Job drawing, mm, ordinate dimensions from the low corner. One solid piece. A direction names the side the tool comes from. Coordinates: 2 decimals unless noted, no trailing zeros. Write each loop counter-clockwise with the first axis right and the second up, starting at its lowest first coordinate (ties: lowest second). Pieces come first, ordered by that corner, then holes.
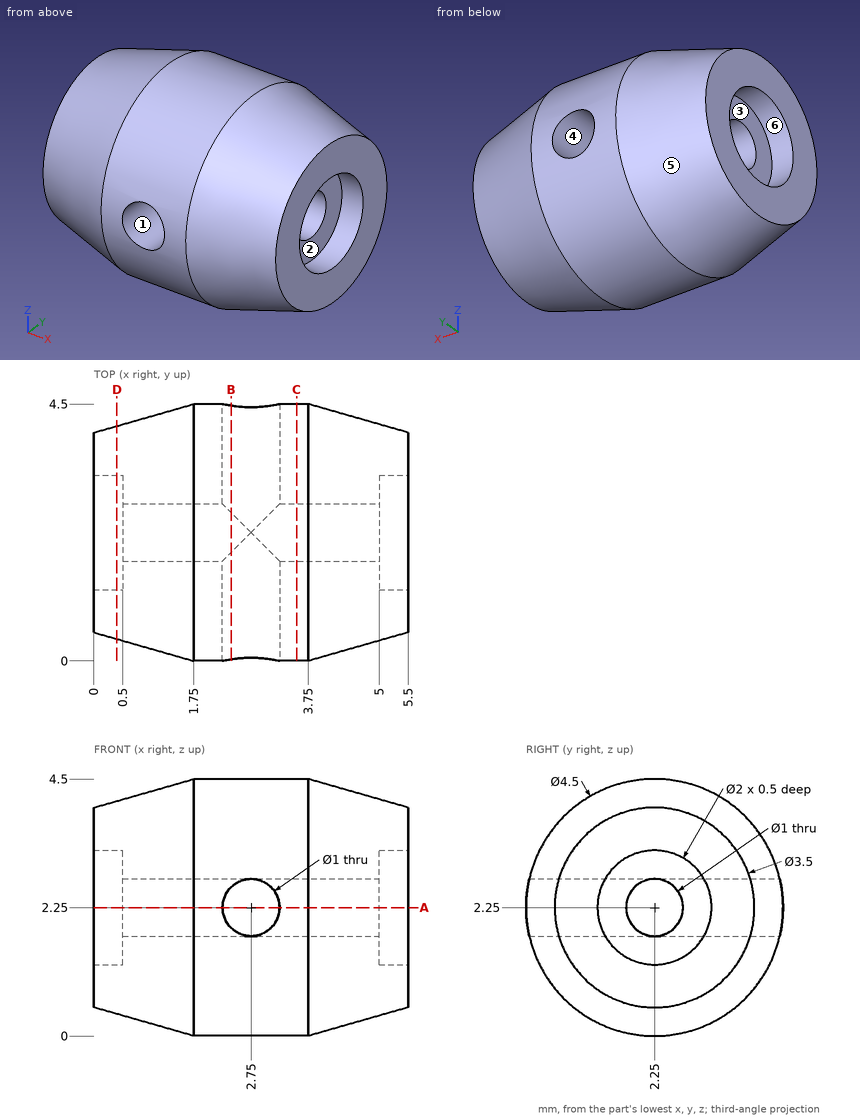
1. Saw through at A-A on z = 2.25. List the corners of the cut face in (x, y), plus the area to 3 significant figures.
Computed values:
outline: (0, 0.5) - (1.75, 0) - (2.25, 0) - (2.25, 1.75) - (0.5, 1.75) - (0.5, 1.25) - (0, 1.25) - close; (0, 3.25) - (0.5, 3.25) - (0.5, 2.75) - (2.25, 2.75) - (2.25, 4.5) - (1.75, 4.5) - (0, 4) - close; (3.25, 0) - (3.75, 0) - (5.5, 0.5) - (5.5, 1.25) - (5, 1.25) - (5, 1.75) - (3.25, 1.75) - close; (3.25, 2.75) - (5, 2.75) - (5, 3.25) - (5.5, 3.25) - (5.5, 4) - (3.75, 4.5) - (3.25, 4.5) - close
area: 13.0 mm2
2. Saw through at C-C on x = 3.55. List the corners of the cut face in (y, z), plus the area to 3 significant figures.
Computed values:
outline: circle Ø4.5 at (2.25, 2.25); hole circle Ø1 at (2.25, 2.25)
area: 15.1 mm2
3. Flat gauge pins, fed straight in: pin 1 (1.2 mm diameter, centred on y = 2.25, z = 2.25, fed in from +X); pin 2 (0.6 mm diameter, centred on y = 2, z = 2, fed in from -X); pin 3 (1.5 mm diameter, centred on x = 3.5, y = 4, fed in from -Z). Where does each tip first touch, or does it go through?
Computed values:
pin 1: stops at x = 5
pin 2: stops at x = 0.5
pin 3: stops at z = 0.23
4. Mould opens along Y. For the marked faces 4, 5 and 6 say: +Y half, -Y half, draft (parallel to the pull), parting line (faces both ways), or undercut.
Computed values:
face 4: draft
face 5: parting line
face 6: undercut
5. Saw through at D-D on x = 0.4. List the corners of the cut face in (y, z), plus the area to 3 significant figures.
Computed values:
outline: circle Ø3.73 at (2.25, 2.25); hole circle Ø2 at (2.25, 2.25)
area: 7.78 mm2
6. Probe line 1 along X through (y, z) = (2.3, 2.9); line 2 along Y through (x, z) = (5.2, 2.25); line 3 along Z through (x, y) = (2.75, 3.9). List the from-to ranges inside material, lowest first.
Computed values:
line 1: x = 0.5 to 5
line 2: y = 0.41 to 1.25, 3.25 to 4.09
line 3: z = 0.72 to 1.75, 2.75 to 3.78
7. Saw through at B-B on x = 2.4. List the corners of the cut face in (y, z).
Computed values:
outline: (0.03, 1.89) arc R2.25 ccw to (4.47, 1.89) - (2.6, 1.89) arc R0.5 cw to (1.9, 1.89) - close; (0.03, 2.61) - (1.9, 2.61) arc R0.5 cw to (2.6, 2.61) - (4.47, 2.61) arc R2.25 ccw to start
8. 3-axis set-ups, long thin cutter, end or side, ignore diameter. For the marked faces 1, 2 and 3: which of +Z, -Z, +X, -X, +Y, -Y reach the whole face in a straight line?
Computed values:
face 1: +Y, -Y
face 2: +X
face 3: -X
